Check sheet for the drawn part. Datum: minimum x, y, z corner. Units: mm. Round coordinates to 2 decimals unless told otherwise and drop trailing zeros. Loops run counter-clockwise (first coordinate to the right, second up) from the corner with the lowest first, then second, coordinate; pieces in that order, holes last.
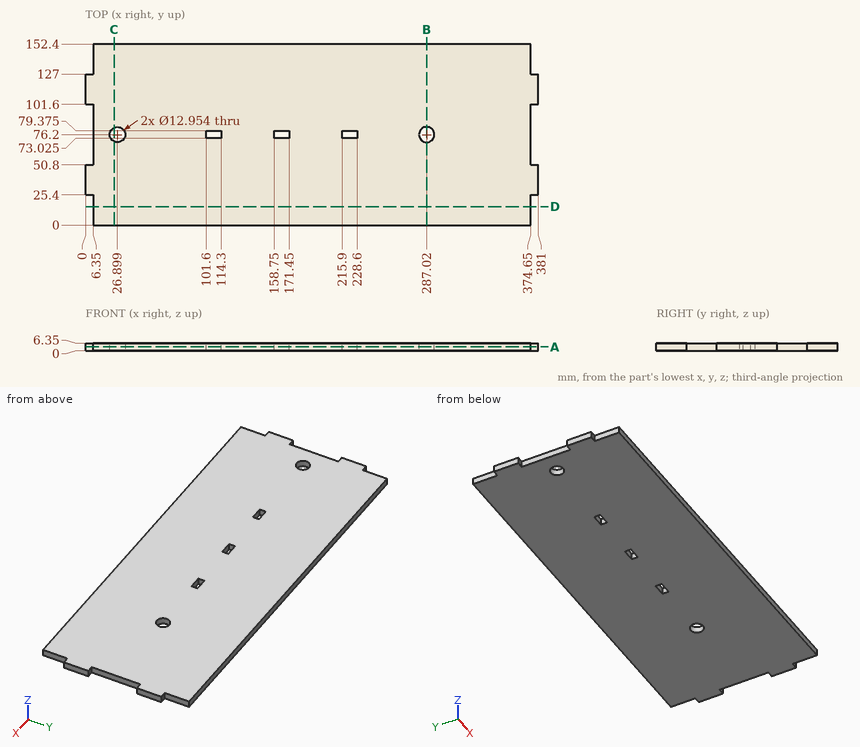
1) Sectioned sample at C-C, the plane x = 24. Record the cut outline in (y, z), then the cut area to 3 significant figures.
Report:
outline: (0, 0) - (70.41, 0) - (70.41, 6.35) - (0, 6.35) - close; (81.99, 0) - (152.4, 0) - (152.4, 6.35) - (81.99, 6.35) - close
area: 894 mm2
2) Sectioned sample at B-B, the plane x = 287.02. Record the cut outline in (y, z).
Report:
outline: (0, 0) - (69.72, 0) - (69.72, 6.35) - (0, 6.35) - close; (82.68, 0) - (152.4, 0) - (152.4, 6.35) - (82.68, 6.35) - close
3) Scan lines: line 1 along Y through (x, z) = (287.02, 2.25); line 2 along Y through (x, z) = (164, 5.75) (1 decimal); line 3 along X through (y, z) = (94.5, 4.25). Record each from-to range of solid material in increasing order.
Report:
line 1: y = 0 to 69.72, 82.68 to 152.4
line 2: y = 0 to 73, 79.4 to 152.4
line 3: x = 6.35 to 374.65
4) Gauge pin test, flat ends, axial feed: pin 1 (1.9 mm diameter, centred on y = 133.5, z = 3.5, fed in from +X); pin 2 (1.9 mm diameter, centred on y = 77.5, z = 4.5, fed in from -X); pin 3 (3 mm diameter, centred on x = 2.5, z = 4.5, fed in from -Y); pin 4 (17 mm diameter, centred on x = 287.02, y = 76.2, fed in from -Z). Record the tip position at first contact, or that the pin passes through.
Report:
pin 1: stops at x = 374.65
pin 2: stops at x = 6.35
pin 3: stops at y = 25.4
pin 4: stops at z = 0
5) Sectioned sample at A-A, the plane z = 3.25. State how many separate pieces and enclosed holes the cut face has, then the cut area to 3 significant figures.
Report:
separate pieces: 1
enclosed holes: 5
area: 56,300 mm2
6) Sectioned sample at D-D, the plane y = 15.5. Record the cut outline in (x, z).
Report:
outline: (6.35, 0) - (374.65, 0) - (374.65, 6.35) - (6.35, 6.35) - close
